Could you check a few things on this model? Use its own coordinates, in mm. Face numbers are marked on the shaded views. A direction names the side the tool comes from. Coordinates: 2 decimals unless noted, no trailing zeros. Loops run counter-clockwise (first coordinate to the right, second up) from the corner with the lowest first, then second, coordinate; pieces in that order, holes last. Notation, with made-up numbers: (11.5, 74.5) - (34.5, 74.5) arc R28 ccw to (34.5, 106.5) - close; hole circle Ø4 at (58, -7.75). An arc over 180 degrees is marked (long way). Use CSV: the item, a comma, the result in double quotes.
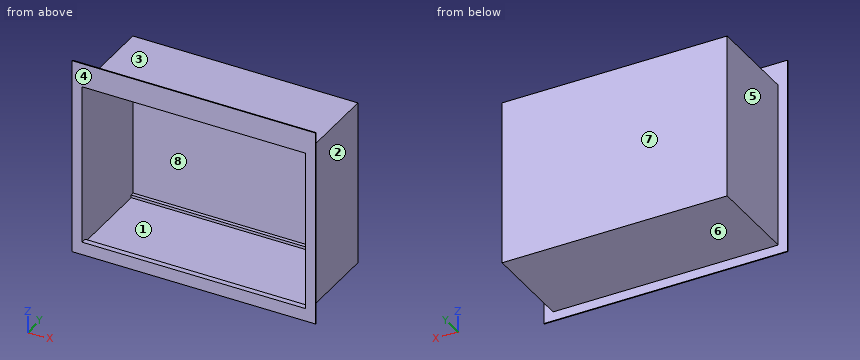
from build123d import *

# Parameters (mm, degrees)
SKETCH_1_W                = 530
SKETCH_1_H                = 430
EXTRUDE_1_DEPTH           = 2
EXTRUDE_1_2_OUTLINE_W     = 490
EXTRUDE_1_2_OUTLINE_H     = 360
EXTRUDE_1_2_DEPTH         = 10
EXTRUDE_START             = 190
EXTRUDE_1_2_2_OUTLINE_W   = 490
EXTRUDE_1_2_2_OUTLINE_H   = 360
EXTRUDE_1_2_2_DEPTH       = 10
EXTRUDE_START_2           = 10
EXTRUDE_1_2_3_OUTLINE_W   = 490
EXTRUDE_1_2_3_OUTLINE_H   = 360
EXTRUDE_1_2_3_OUTLINE_W_2 = 486
EXTRUDE_1_2_3_OUTLINE_H_2 = 356
EXTRUDE_1_2_3_DEPTH       = 180
SKETCH_3_W                = 486
SKETCH_3_H                = 350
CUT_EXTRUDE_1_DEPTH       = 200


# Read off the part's stored shape, not the designer's step: Вытянуть-Тонкостенный1
with BuildPart() as part:
    # Эскиз1 → Extrude 1 (new body)
    with BuildSketch(Plane(origin=(0, 0, 0), x_dir=(1, 0, 0), z_dir=(0, 1, 0))):
        with Locations((265, 215)):
            Rectangle(SKETCH_1_W, SKETCH_1_H)
    extrude(amount=EXTRUDE_1_DEPTH)

    # Extrude 1 2 outline → Extrude 1 2 (add)
    with BuildSketch(Plane(origin=(0, 2, 0), x_dir=(1, 0, 0), z_dir=(0, 1, 0))):
        with Locations((265, 230)):
            Rectangle(EXTRUDE_1_2_OUTLINE_W, EXTRUDE_1_2_OUTLINE_H)
    extrude(amount=EXTRUDE_1_2_DEPTH)



with BuildPart() as body_2:
    # Extrude 1 2 2 outline → Extrude 1 2 2 (new body)
    with BuildSketch(Plane(origin=(0, 2, 0), x_dir=(1, 0, 0), z_dir=(0, 1, 0)).offset(EXTRUDE_START)):
        with Locations((265, 230)):
            Rectangle(EXTRUDE_1_2_2_OUTLINE_W, EXTRUDE_1_2_2_OUTLINE_H)
    extrude(amount=EXTRUDE_1_2_2_DEPTH)


with BuildPart() as part_1:
    add(part.part)

    add(body_2.part)  # Extrude 1 2 3 merges body 2
    # Extrude 1 2 3 outline → Extrude 1 2 3 (add)
    with BuildSketch(Plane(origin=(0, 2, 0), x_dir=(1, 0, 0), z_dir=(0, 1, 0)).offset(EXTRUDE_START_2)):
        with Locations((265, 230)):
            Rectangle(EXTRUDE_1_2_3_OUTLINE_W, EXTRUDE_1_2_3_OUTLINE_H)
        with Locations((265, 230)):
            Rectangle(EXTRUDE_1_2_3_OUTLINE_W_2, EXTRUDE_1_2_3_OUTLINE_H_2, mode=Mode.SUBTRACT)
    extrude(amount=EXTRUDE_1_2_3_DEPTH)

    # Эскиз3 → Вырез-Вытянуть1 (cut)
    with BuildSketch(Plane.XZ):
        with Locations((265, -227)):
            Rectangle(SKETCH_3_W, SKETCH_3_H)
    extrude(amount=-CUT_EXTRUDE_1_DEPTH, mode=Mode.SUBTRACT)


solid = part_1.part
(1) Will these pins go through, and if not, where does the flat tip stop? pin 1 (5 mm diameter, centred on x = 153, y = 148.5, fed in from -Z); pin 2 (12 mm diameter, centred on y = 103.5, z = -191.5, fed in from +X); pin 3 (1.5 mm diameter, centred on x = 366.5, y = 129, fed in from +Z).
Computed:
pin 1,"stops at z = -410"
pin 2,"stops at x = 510"
pin 3,"stops at z = -50"
(2) Suppose I cut it at D-D (z = -33). Write out the boundary of the cut face in (x, y).
Computed:
outline,"(0, 0) - (530, 0) - (530, 2) - (0, 2) - close"
(3) Suppose I cut it at B-B (z = -107). Write out the boundary of the cut face in (x, y).
Computed:
outline,"(0, 0) - (22, 0) - (22, 200) - (508, 200) - (508, 0) - (530, 0) - (530, 2) - (510, 2) - (510, 202) - (20, 202) - (20, 2) - (0, 2) - close"
(4) Thinking about a two-plate mould opening in Z: for the marked faces 6, 7 and 8, which applies, +Z half, -Z half, draft (parallel to the pull), parting line (faces both ways), or undercut?
Computed:
face 6,"-Z half"
face 7,"draft"
face 8,"undercut"
(5) Which directions (+Z, -Z, +X, -X, +Y, -Y) give clear straight access to the entire face, cutting with the end or side of a thin tool? Please do the marked faces 1, 2, 3, 4 and 5.
Computed:
face 1,"none"
face 2,"+Z, -Z, +X, +Y"
face 3,"+Z, +X, -X, +Y"
face 4,"+Z, -Z, +X, -X, -Y"
face 5,"+Z, -Z, -X, +Y"
(6) Please list where these lines run through material, in increasing order: line 1 (X direction, y = 162.5, z = -265.5); line 2 (Z direction, x = 399, y = 112); line 3 (Y direction, x = 228.5, z = -263).
Computed:
line 1,"x = 20 to 22, 508 to 510"
line 2,"z = -410 to -408, -52 to -50"
line 3,"y = 200 to 202"
(7) Suppose I cut it at A-A (x = 330). Write out the boundary of the cut face in (y, z).
Computed:
outline,"(0, -430) - (2, -430) - (2, -410) - (202, -410) - (202, -50) - (2, -50) - (2, 0) - (0, 0) - (0, -52) - (200, -52) - (200, -402) - (192, -402) - (192, -408) - (12, -408) - (12, -402) - (0, -402) - close"
(8) Suppose I cut it at C-C (y = 114). Write out the boundary of the cut face in (x, z), plus the area to 3 significant figures.
Computed:
outline,"(20, -410) - (510, -410) - (510, -50) - (20, -50) - close; hole (22, -408) - (508, -408) - (508, -52) - (22, -52) - close"
area,"3,380 mm²"
